Check sheet for the drawn part. Datum: minimum x, y, z corner. Units: mm. A direction names the side the tool comes from. Give positions to 0.01 mm unless a question says otherwise; leave off trailing zeros. Order: outer loops, then holes, each group sorted by start corner. A loop starts at its lowest first (then second) coordinate and runs counter-clockwise, first axis right, second up.
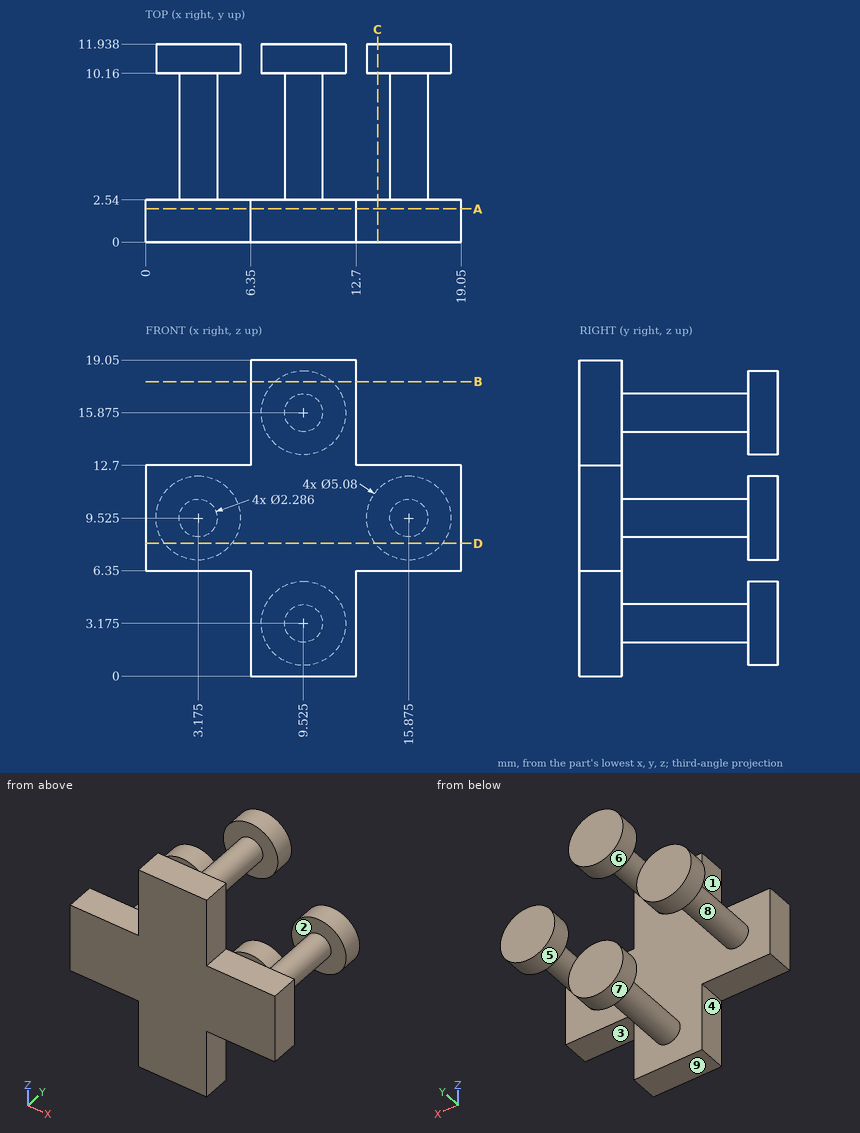
Q1. Go/stop test with flat-tipped pins: P1, Ø5, axis at x = 2, y = 3.5, coming from the -Z side; P2, Ø3, axis at y = 6, z = 6, coming from the +X side; P3, Ø4, axis at y = 7.5, z = 11, coming from the +X side; P4, Ø2, axis at x = 3, y = 1, coming from the +Z side. Record where each tip stops, or that it passes through.
Q2. Sectioned sample at B-B, the plane z = 17.75. Record the cut outline in (x, y), plus the area to 3 significant figures.
Q3. Sectioned sample at C-C, the plane x = 14. Record the cut outline in (y, z).
Q4. Tool access check on the marked faces 1, 2, 3, 4 and 5. Record the directions out of +Z, -Z, +X, -X, +Y, -Y that give a thin tool (end or side, any length) a straight path to the whole face; none if there is none.
Q5. Sectioned sample at A-A, the plane y = 2. Record the cut outline in (x, z).
Q6. Material ranges on line 1 (Y direction, x = 4.5, z = 8); line 2 (Z direction, x = 3.5, y = 2.5); line 3 (Z direction, x = 9.5, y = 5), recorded low to high.
Q7. Draft check along Z on the marked faces 6, 7, 8 and 9. Enter one of: pulls with the +Z half, pulls with the -Z half, needs draft (parallel to the pull), parting line crosses it, or undercut.
Q8. Sectioned sample at D-D, the plane z = 8. Record the cut outline in (x, y), plus the area to 3 significant figures.
Filled in:
1. P1: stops at z = 6.35
1. P2: passes through
1. P3: stops at x = 17.02
1. P4: stops at z = 12.7
2. outline: (6.35, 0) - (12.7, 0) - (12.7, 2.54) - (6.35, 2.54) - close; (7.81, 10.16) - (11.24, 10.16) - (11.24, 11.94) - (7.81, 11.94) - close
2. area: 22.2 mm2
3. outline: (0, 6.35) - (2.54, 6.35) - (2.54, 12.7) - (0, 12.7) - close; (10.16, 7.81) - (11.94, 7.81) - (11.94, 11.24) - (10.16, 11.24) - close
4. face 1: +Z, -X, +Y, -Y
4. face 2: none
4. face 3: -Z, +X, +Y, -Y
4. face 4: -Z, -X, +Y, -Y
4. face 5: +Y
5. outline: (0, 6.35) - (6.35, 6.35) - (6.35, 0) - (12.7, 0) - (12.7, 6.35) - (19.05, 6.35) - (19.05, 12.7) - (12.7, 12.7) - (12.7, 19.05) - (6.35, 19.05) - (6.35, 12.7) - (0, 12.7) - close
6. line 1: y = 0 to 2.54, 10.16 to 11.94
6. line 2: z = 6.35 to 12.7
6. line 3: z = 2.03 to 4.32, 14.73 to 17.02
7. face 6: undercut
7. face 7: undercut
7. face 8: parting line crosses it
7. face 9: pulls with the -Z half
8. outline: (0, 0) - (19.05, 0) - (19.05, 2.54) - (0, 2.54) - close; (1.14, 10.16) - (5.21, 10.16) - (5.21, 11.94) - (1.14, 11.94) - close; (13.84, 10.16) - (17.91, 10.16) - (17.91, 11.94) - (13.84, 11.94) - close
8. area: 62.8 mm2
